Answer from the drawing. Dimensions are ordinates in mm from the lowest x, y and z of the part. A direction names the side the tool comes from. Coordinates: 2 decimals unless noted, no trailing zeros. Loops run counter-clockwise (first coordinate to the right, second up) from the corner with the lowest first, then second, coordinate; pieces in that order, holes last.
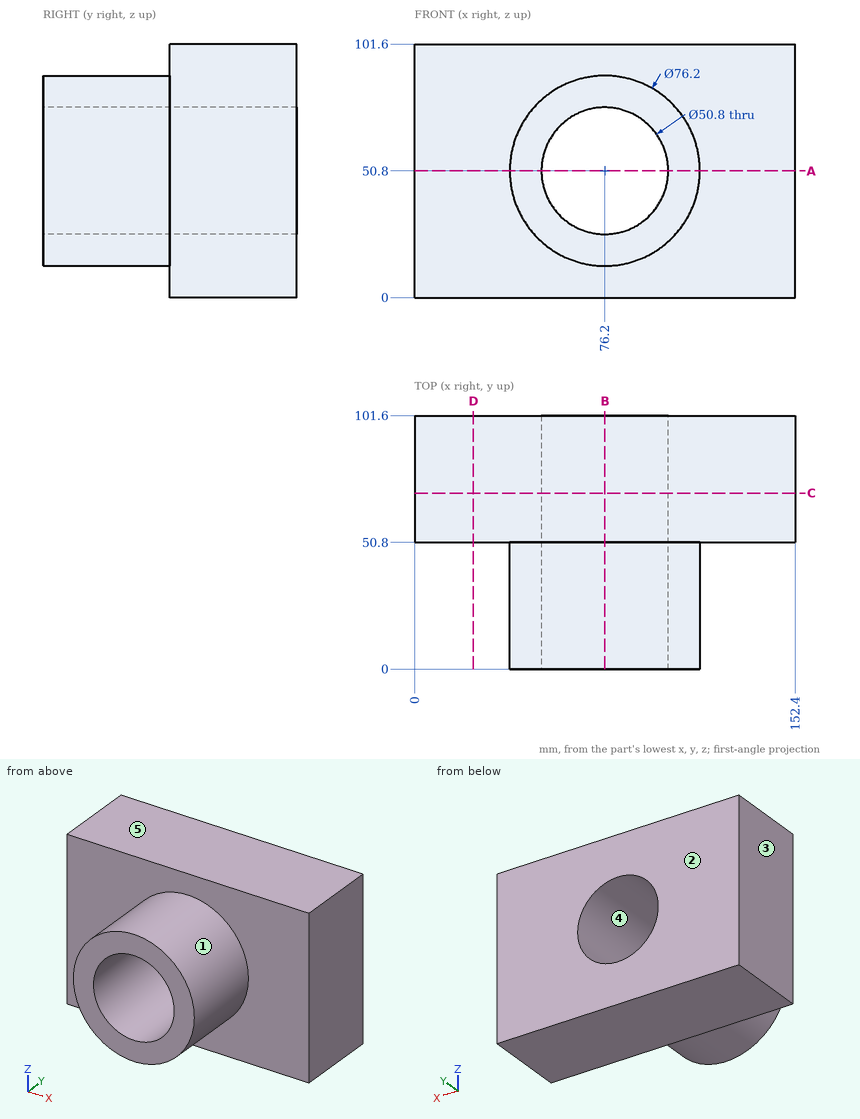
Item 1: Which of the six approach directions +Z, -Z, +X, -X, +Y, -Y give full straight-line access (tool end or side, diameter ignored) to the marked faces 1 and 2?
Numbers:
face 1: -Y
face 2: +Z, -Z, +X, -X, +Y
Item 2: Given pin 1 (4 mm diameter, centred on x = 23.5, z = 40, fed in from -Y); pin 2 (10 mm diameter, centred on x = 47.5, y = 23.5, fed in from +Z), each flat-ended and moving along its own axis, determine where each tip first touches the part or whether it passes through.
Numbers:
pin 1: stops at y = 50.8
pin 2: stops at z = 80.63
Item 3: Determine the mould class of the marked faces 3, 4 and 5 for opening direction Z: released by +Z, released by -Z, zero draft, split by the parting line, or undercut.
Numbers:
face 3: zero draft
face 4: undercut
face 5: released by +Z
Item 4: A cutting plane is placed at C-C on y = 70.5. Determine the outline of the cut face in (x, z), then the cut area to 3 significant figures.
Numbers:
outline: (0, 0) - (152.4, 0) - (152.4, 101.6) - (0, 101.6) - close; hole circle Ø50.8 at (76.2, 50.8)
area: 13,500 mm2
Item 5: A cutting plane is placed at B-B on x = 76.2. Determine the outline of the cut face in (y, z), then the cut area to 3 significant figures.
Numbers:
outline: (0, 12.7) - (50.8, 12.7) - (50.8, 0) - (101.6, 0) - (101.6, 25.4) - (0, 25.4) - close; (0, 76.2) - (101.6, 76.2) - (101.6, 101.6) - (50.8, 101.6) - (50.8, 88.9) - (0, 88.9) - close
area: 3,870 mm2
Item 6: A cutting plane is placed at A-A on z = 50.8. Determine the outline of the cut face in (x, y).
Numbers:
outline: (0, 50.8) - (38.1, 50.8) - (38.1, 0) - (50.8, 0) - (50.8, 101.6) - (0, 101.6) - close; (101.6, 0) - (114.3, 0) - (114.3, 50.8) - (152.4, 50.8) - (152.4, 101.6) - (101.6, 101.6) - close
Item 7: A cutting plane is placed at D-D on x = 23.5. Determine the outline of the cut face in (y, z).
Numbers:
outline: (50.8, 0) - (101.6, 0) - (101.6, 101.6) - (50.8, 101.6) - close
Item 8: Find the intervals of material crossed by line 1 along Z through (x, y) = (76.2, 40); line 2 along X through (y, z) = (42, 50); line 3 along Z through (x, y) = (76.2, 63), in increasing order.
Numbers:
line 1: z = 12.7 to 25.4, 76.2 to 88.9
line 2: x = 38.11 to 50.81, 101.59 to 114.29
line 3: z = 0 to 25.4, 76.2 to 101.6
